Geometry check sheet. Reference: the model listing, model coordinates, mm. Face numbers are marked on the shaded views. A direction names the side the tool comes from. Coordinates: 2 decimals unless noted, no trailing zeros. Write each loop counter-clockwise with the first axis right and the second up, starting at its lowest first coordinate (ties: lowest second). Pieces come first, ordered by that corner, then holes. Notation, with made-up numbers: M -16,42.25 L 30,42.25 A18 cw 30,59.25 Z; hole C 8.5,65 d2. An arc over 180 degrees is marked long. Write each question's results on one line, items separated by ' | '.
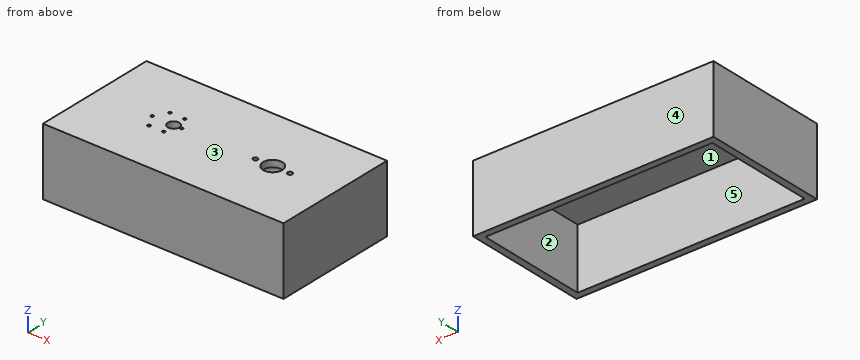
```python
from build123d import *

# Parameters (mm, degrees)
SKETCH1_W           = 250
SKETCH1_H           = 130
BOSS_EXTRUDE1_DEPTH = 70
SHELL1_T            = -7
SKETCH2_R           = 10
SKETCH2_R_2         = 2.5
SKETCH2_R_3         = 1.5
SKETCH2_R_4         = 6
CUT_EXTRUDE1_DEPTH  = 90


with BuildPart() as part:
    # Sketch1 → Boss-Extrude1 (new body)
    with BuildSketch(Plane.XY):
        Rectangle(SKETCH1_W, SKETCH1_H)
    extrude(amount=BOSS_EXTRUDE1_DEPTH)

    # Shell1
    shell1_openings = [part.faces().sort_by_distance(p)[0] for p in [
        (0, 0, 0),
    ]]
    offset(amount=SHELL1_T, openings=shell1_openings, kind=Kind.INTERSECTION)

    # Sketch2 → Cut-Extrude1 (cut)
    with BuildSketch(Plane.XY.offset(70)):
        with Locations((60, 0)):
            Circle(SKETCH2_R)
        with Locations((42, 0)):
            Circle(SKETCH2_R_2)
        with Locations((78, 0)):
            Circle(SKETCH2_R_2)
        with Locations((-34.7, 0)):
            Circle(SKETCH2_R_3)
        with Locations((-42.35, -13.250188678)):
            Circle(SKETCH2_R_3)
        with Locations((-57.65, -13.250188678)):
            Circle(SKETCH2_R_3)
        with Locations((-65.3, 0)):
            Circle(SKETCH2_R_3)
        with Locations((-57.65, 13.250188678)):
            Circle(SKETCH2_R_3)
        with Locations((-42.35, 13.250188678)):
            Circle(SKETCH2_R_3)
        with Locations((-43, 0)):
            Circle(SKETCH2_R_4)
    extrude(amount=-CUT_EXTRUDE1_DEPTH, mode=Mode.SUBTRACT)


solid = part.part
```
Q1. Sectioned sample at D-D on x = -53.5. Record the cut outline in (y, z), and give its area (3 significant figures).
Geometry check:
outline: M -65,0 L -58,0 L -58,63 L 58,63 L 58,0 L 65,0 L 65,70 L -65,70 Z | area: 1,790 mm2
Q2. Sectioned sample at C-C on y = 41. Record the cut outline in (x, z).
Geometry check:
outline: M -125,0 L -118,0 L -118,63 L 118,63 L 118,0 L 125,0 L 125,70 L -125,70 Z
Q3. Mould release check, pull along Z, two halves, no side actions. Record for the marked faces 1, 2 and 3: pulls with the +Z half, pulls with the -Z half, needs draft (parallel to the pull), parting line crosses it, or undercut.
Geometry check:
face 1: pulls with the -Z half | face 2: needs draft | face 3: pulls with the +Z half
Q4. Depth check by flat-ended pin: P1, Ø1.8, axis at x = -65.3, y = 0, coming from the +Z side. Enter the tip coordinate at first touch or a pass-through.
Geometry check:
P1: passes through
Q5. Scan lines: probe 1 along Y at (x, z) = (60, 17.5); probe 2 along X at (y, z) = (50.5, 27.5); probe 3 along Y at (x, z) = (42, 68). Record each from-to range of solid material in increasing order.
Geometry check:
probe 1: y = -65 to -58, 58 to 65 | probe 2: x = -125 to -118, 118 to 125 | probe 3: y = -65 to -2.5, 2.5 to 65
Q6. Sectioned sample at A-A on z = 46. Record the cut outline in (x, y).
Geometry check:
outline: M -125,-65 L 125,-65 L 125,65 L -125,65 Z; hole M -118,-58 L 118,-58 L 118,58 L -118,58 Z
Q7. Access from +Z, -Z, +X, -X, +Y, -Y to the whole of each face (thin tool, end or side, straight path). Record for the marked faces 4 and 5.
Geometry check:
face 4: +Z, -Z, +X, -X, +Y | face 5: -Z
Q8. Sectioned sample at B-B on x = 78. Record the cut outline in (y, z).
Geometry check:
outline: M -65,0 L -58,0 L -58,63 L -2.5,63 L -2.5,70 L -65,70 Z; M 2.5,63 L 58,63 L 58,0 L 65,0 L 65,70 L 2.5,70 Z
